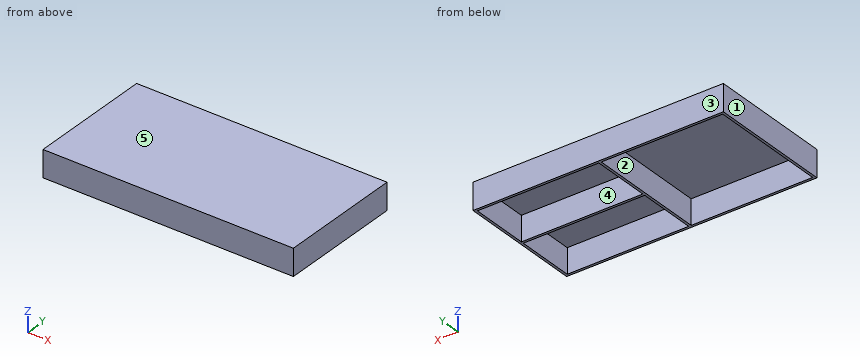
Autodesk Inventor part; units mm, degrees
ref_plane "YZ Plane" through (0, 0, 0) normal (1, 0, 0) x (0, 1, 0)
ref_plane "XZ Plane" through (0, 0, 0) normal (0, 1, 0) x (-1, 0, 0)
ref_plane "XY Plane" through (0, 0, 0) normal (0, 0, 1) x (1, 0, 0)
sketch "Esboço1" plane through (0, 0, 0) normal (0, 0, 1) x (1, 0, 0)
  line L0 (-150, -75) -> (150, -75)
  line L1 (150, -75) -> (150, 75)
  line L2 (150, 75) -> (-150, 75)
  line L3 (-150, 75) -> (-150, -75)
  line L4 (-150, -75) -> (150, 75) construction
  line L5 (-147, 72) -> (147, 72)
  line L6 (147, 72) -> (147, -72)
  line L7 (147, -72) -> (-147, -72)
  line L8 (-147, -72) -> (-147, 72)
  line L9 (0, 72) -> (0, 0) construction
  line L10 (147, 0) -> (0, 0) construction
  line L11 (1.5, 72) -> (1.5, 1.5)
  line L12 (1.5, 1.5) -> (147, 1.5)
  line L13 (0, 0) -> (0, -72) construction
  line L14 (147, -1.5) -> (1.5, -1.5)
  line L15 (1.5, -1.5) -> (1.5, -72)
  line L16 (150, -75) -> (144, -72) construction
  line L17 (0, 0) -> (-150, 75) construction
  line L18 (-1.5, 72) -> (-1.5, 0)
  line L19 (-1.5, 0) -> (-1.5, -72)
  dimension "d0" = 150
  dimension "d1" = 300
  dimension "d2" = 3
  dimension "d3" = 1.5
  dimension "d5" = 1.5
  dimension "d6" = 1.5
  dimension "d7" = 1.5
extrude "Extrusão1" add sketch "Esboço1" along normal blind 2 contours L3 L2 L1 L0 | L5 L18 L19 L7 L8 | L5 L11 L12 L6 L14 L15 L7 L19 L18 | L5 L6 L12 L11 | L15 L14 L6 L7
extrude "Extrusão2" add sketch "Esboço1" against normal blind 30 contours L3 L2 L1 L0 | L5 L11 L12 L6 L14 L15 L7 L19 L18
sketch "Esboço2" plane through (150, -75, 2) normal (1, 0, 0) x (0, 0, -1)
  point P0 (2, 75)
properties part number "nsabo"
Check sheet for the modelled part. Datum: model origin and axes. Units: mm. Face numbers are marked on the shaded views. A direction names the side the tool comes from. Round coordinates to 2 decimals unless told otherwise and drop trailing zeros. Order: outer loops, then holes, each group sorted by start corner. A loop starts at its lowest first (then second) coordinate and runs counter-clockwise, first axis right, second up. Notation, with made-up numbers: (57.25, -11) - (93.25, -11) arc R27 cw to (93.25, 16) - close; hole circle Ø9 at (-27.75, 17). An arc over 180 degrees is marked (long way). Answer as CSV lines item,"result". Start each with the question number.
1) Section check C-C (z = -4.5). Record the cut outline in (x, y).
2) Section check D-D (x = -91). Record the cut outline in (y, z).
3) Scan lines: probe 1 along X at (y, z) = (68, -21); probe 2 along Y at (x, z) = (80.5, -25.5); probe 3 along Y at (x, z) = (-125.5, -14.5). Record each from-to range of solid material in increasing order.
4) Tool access check on the marked faces 4 and 5. Record the directions out of +Z, -Z, +X, -X, +Y, -Y that give a thin tool (end or side, any length) a straight path to the whole face; none if there is none.
5) Draft check along X on the marked faces 1, 2 and 3. Enter one of: +X half, -X half, draft (parallel to the pull), parting line (faces both ways), or undercut.
6) Depth check by flat-ended pin: pin 1 (21 mm diameter, centred on x = 100, y = 49, fed in from -Z). Enter the tip coordinate at first touch or a pass-through.
7) Section check A-A (x = 73.5). Record the cut outline in (y, z), then the cut area to 3 significant figures.
8) Section check B-B (y = 50.5). Record the cut outline in (x, z).
Determined:
1,outline,"(-150, -75) - (150, -75) - (150, 75) - (-150, 75) - close; hole (-147, -72) - (-1.5, -72) - (-1.5, 72) - (-147, 72) - close; hole (1.5, -72) - (147, -72) - (147, -1.5) - (1.5, -1.5) - close; hole (1.5, 1.5) - (147, 1.5) - (147, 72) - (1.5, 72) - close"
2,outline,"(-75, -30) - (-72, -30) - (-72, 0) - (72, 0) - (72, -30) - (75, -30) - (75, 2) - (-75, 2) - close"
3,probe 1,"-150 to -147, -1.5 to 1.5, 147 to 150"
3,probe 2,"-75 to -72, -1.5 to 1.5, 72 to 75"
3,probe 3,"-75 to -72, 72 to 75"
4,face 4,"-Z"
4,face 5,"+Z, +X, -X, +Y, -Y"
5,face 1,"-X half"
5,face 2,"undercut"
5,face 3,"draft"
6,pin 1,"z = 0"
7,outline,"(-75, -30) - (-72, -30) - (-72, 0) - (-1.5, 0) - (-1.5, -30) - (1.5, -30) - (1.5, 0) - (72, 0) - (72, -30) - (75, -30) - (75, 2) - (-75, 2) - close"
7,area,"570 mm^2"
8,outline,"(-150, -30) - (-147, -30) - (-147, 0) - (-1.5, 0) - (-1.5, -30) - (1.5, -30) - (1.5, 0) - (147, 0) - (147, -30) - (150, -30) - (150, 2) - (-150, 2) - close"
